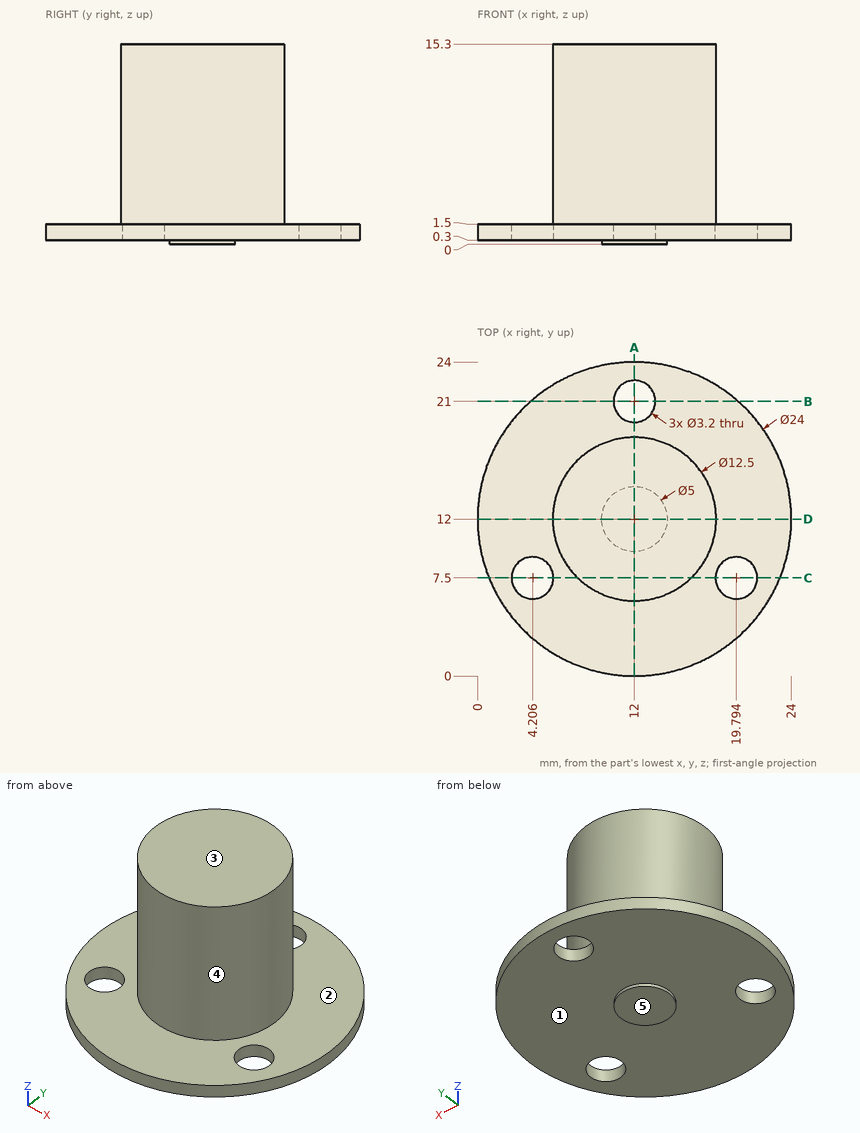
Design review of the part shown in the three views and the two pictorial views. Dimensions are in mm from the part's minimum x, y and z. A direction names the side the tool comes from. Coordinates: 2 decimals unless noted, no trailing zeros. Order: outer loops, then holes, each group sorted by start corner. A loop starts at its lowest first (then second) coordinate and runs counter-clockwise, first axis right, second up. Notation, with made-up numbers: (7.25, -2) - (21.25, -2) arc R22 cw to (21.25, 5) - close; hole circle Ø6 at (28, 65.25). An arc over 180 degrees is marked (long way). One line per question, with ' | ' between items.
Q1. Consider section B-B, the plane y = 21. Give the boundary of the cut face in (x, z), then the cut area to 3 significant figures.
Answer key:
outline: (4.06, 0.3) - (10.4, 0.3) - (10.4, 1.5) - (4.06, 1.5) - close; (13.6, 0.3) - (19.94, 0.3) - (19.94, 1.5) - (13.6, 1.5) - close | area: 15.2 mm2
Q2. Consider section A-A, the plane x = 12. Give the boundary of the cut face in (y, z), then the cut area to 3 significant figures.
Answer key:
outline: (0, 0.3) - (9.5, 0.3) - (9.5, 0) - (14.5, 0) - (14.5, 0.3) - (19.4, 0.3) - (19.4, 1.5) - (18.25, 1.5) - (18.25, 15.3) - (5.75, 15.3) - (5.75, 1.5) - (0, 1.5) - close; (22.6, 0.3) - (24, 0.3) - (24, 1.5) - (22.6, 1.5) - close | area: 199 mm2
Q3. The part is to be moulded in two halves that separate along Z. For the marked faces 3, 4 and 5, say which applies: +Z half, -Z half, draft (parallel to the pull), parting line (faces both ways), or undercut.
Answer key:
face 3: +Z half | face 4: draft | face 5: -Z half
Q4. Clearance check with flat-ended pins moving along their axes: pin 1 Ø1.5 at (x, z) = (5.5, 3.5) entering from -Y; pin 2 Ø8 at (y, z) = (20.5, 10) entering from +X; pin 3 Ø8 at (y, z) = (19, 10) entering from -X; pin 4 Ø2.5 at (x, y) = (19.79, 7.5) entering from -Z. State where each tip first meets the part, or that it passes through.
Answer key:
pin 1: stops at y = 9.55 | pin 2: stops at x = 16.34 | pin 3: stops at x = 6.52 | pin 4: passes through
Q5. To check wall thickness, follow line 1 along Z through (x, y) = (16, 10.5); line 2 along Z through (x, y) = (5, 11.5); line 3 along Y through (x, z) = (11.75, 8.5) (3 decimals). State the ranges of each line that lie inside material, in increasing order.
Answer key:
line 1: z = 0.3 to 15.3 | line 2: z = 0.3 to 1.5 | line 3: y = 5.755 to 18.245
Q6. Consider section C-C, the plane y = 7.5. Give the boundary of the cut face in (x, z).
Answer key:
outline: (0.88, 0.3) - (2.61, 0.3) - (2.61, 1.5) - (0.88, 1.5) - close; (5.81, 0.3) - (18.19, 0.3) - (18.19, 1.5) - (16.34, 1.5) - (16.34, 15.3) - (7.66, 15.3) - (7.66, 1.5) - (5.81, 1.5) - close; (21.39, 0.3) - (23.12, 0.3) - (23.12, 1.5) - (21.39, 1.5) - close
Q7. Consider section D-D, the plane y = 12. Give the boundary of the cut face in (x, z).
Answer key:
outline: (0, 0.3) - (9.5, 0.3) - (9.5, 0) - (14.5, 0) - (14.5, 0.3) - (24, 0.3) - (24, 1.5) - (18.25, 1.5) - (18.25, 15.3) - (5.75, 15.3) - (5.75, 1.5) - (0, 1.5) - close
Q8. For the marked faces 1 and 2, list the 3-axis set-ups (+Z, -Z, +X, -X, +Y, -Y) from which the entire face can be reached by the end or side of a thin tool; tool diameter is ignored.
Answer key:
face 1: -Z | face 2: +Z
